Autodesk Inventor part; units mm, degrees
ref_plane "Plano inicial" through (0, 0, 35) normal (0, 0, 1) x (1, 0, 0)
ref_plane "Plano final" through (0, 0, 465) normal (0, 0, 1) x (1, 0, 0)
ref_plane "Plano de trabajo4" through (-640, 29, 465) normal (0, 0, 1) x (1, 0, 0)
ref_plane "Plano inicial" through (0, 0, 35) normal (0, 0, 1) x (1, 0, 0)
ref_plane "Plano final" through (0, 0, 465) normal (0, 0, 1) x (1, 0, 0)
sketch "Boceto" plane through (0, 0, 0) normal (0, 0, 1) x (1, 0, 0)
  line L0 (-25, -21) -> (-25, 21)
  line L1 (-21, 25) -> (21, 25)
  line L2 (25, 21) -> (25, -21)
  line L3 (21, -25) -> (-21, -25)
  arc A0 (-25, -21) -> (-21, -25) centre (-21, -21) ccw
  arc A1 (25, 21) -> (21, 25) centre (21, 21) ccw
  arc A2 (-21, 25) -> (-25, 21) centre (-21, 21) ccw
  arc A3 (21, -25) -> (25, -21) centre (21, -21) ccw
  arc A4 (-21, 23) -> (-23, 21) centre (-21, 21) ccw
  line L4 (-21, 23) -> (21, 23)
  arc A5 (23, 21) -> (21, 23) centre (21, 21) ccw
  line L5 (23, 21) -> (23, -21)
  arc A6 (21, -23) -> (23, -21) centre (21, -21) ccw
  line L6 (21, -23) -> (-21, -23)
  arc A7 (-23, -21) -> (-21, -23) centre (-21, -21) ccw
  line L7 (-23, -21) -> (-23, 21)
  line L8 (0, 36.1598) -> (0, -36.1598) construction
  line L9 (-36.1598, 0) -> (36.1598, 0) construction
  dimension "d7" = 4
  dimension "d9" = 50
  dimension "d11" = 50
  dimension "d12" = 2
  dimension "d15" = 25
  dimension "d16" = 25
extrude "Cuerpo" add sketch "Boceto" along normal up to surface (430 mm away) from surface at 35
sketch "Sketch3" plane through (0, 0, 0) normal (0, 0, 1) x (1, 0, 0)
  line L0 (0, 0) -> (10, 0)
ref_plane "Work Plane3" through (0, 0, 0) normal (0, -1, 0) x (1, 0, 0)
sketch "Sketch4" plane through (0, 0, 0) normal (0, -1, 0) x (1, 0, 0)
  line L0 (-2, 35) -> (12, 35)
  line L1 (-2, 465) -> (12, 465)
  dimension "d18" = 430
ref_plane "Plano de trabajo4" through (-640, 29, 465) normal (0, 0, 1) x (1, 0, 0)
split "Dividir1" plane through (-640, 29, 465) removes the side toward (0, 0, 1)
ref_plane "Plano de trabajo5" through (-640, -29, 35) normal (0, 0, -1) x (-1, 0, 0)
split "Dividir2" plane through (-640, -29, 35) removes the side toward (0, 0, -1)
equation "\"d7\" = G_IR"
equation "\"d9\" = G_W"
equation "\"d11\" = G_H"
equation "\"d12\" = G_T"
equation "\"d15\" = 0.5 * d9"
equation "\"d16\" = 0.5 * d11"
equation "\"d3\" = G_L"
equation "\"G_W\" = 50"
equation "\"G_H\" = 50"
equation "\"G_T\" = 2"
equation "\"G_IR\" = 4"
equation "\"G_L\" = d18"
equation "\"G_OFFSET_START\" = -35"
equation "\"G_OFFSET_END\" = -35"
equation "\"d13\" = -G_OFFSET_START"
equation "\"d14\" = G_OFFSET_END + B_L"
properties part number "ISO 10799-2 - 50x50x2 - 430" material "Galvanizado catalogo 1"
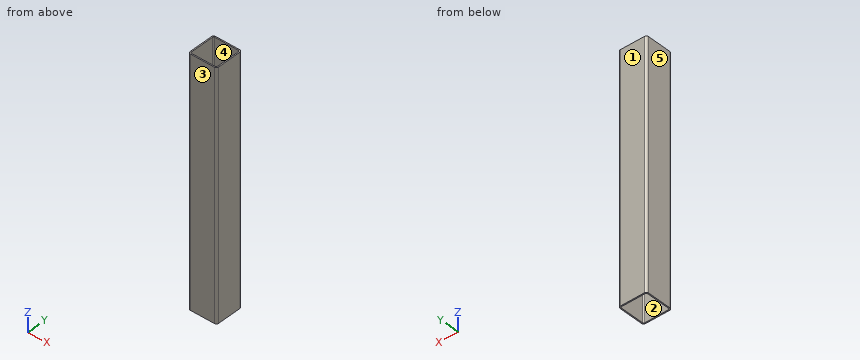
Input: part model. Units: mm. Frame: model coordinates. Face numbers are marked on the shaded views. A direction names the side the tool comes from. Round coordinates to 2 decimals unless told otherwise and drop trailing zeros. Order: outer loops, then holes, each group sorted by start corner. A loop starts at its lowest first (then second) coordinate and runs counter-clockwise, first axis right, second up. Notation, with made-up numbers: (9.25, -32.5) - (43.25, -32.5) arc R21 ccw to (43.25, -9.5) - close; hole circle Ø11 at (-15.75, 25). An arc over 180 degrees is marked (long way). Use a Markdown table: item, result.
1. Section B-B on z = 212. Return the cut outline in (x, y).
Evaluation:
| item | result |
|---|---|
| outline | (-25, -21) arc R4 ccw to (-21, -25) - (21, -25) arc R4 ccw to (25, -21) - (25, 21) arc R4 ccw to (21, 25) - (-21, 25) arc R4 ccw to (-25, 21) - close; hole (-23, -21) arc R2 ccw to (-21, -23) - (21, -23) arc R2 ccw to (23, -21) - (23, 21) arc R2 ccw to (21, 23) - (-21, 23) arc R2 ccw to (-23, 21) - close |
2. Material intervals for probe 1 along Y at (x, z) = (2.5, 88); probe 2 along Y at (x, z) = (23.5, 114), sorted ascending.
Evaluation:
| item | result |
|---|---|
| probe 1 | -25 to -23, 23 to 25 |
| probe 2 | -24.12 to 24.12 |
3. Section A-A on x = 6. Return the cut outline in (y, z).
Evaluation:
| item | result |
|---|---|
| outline | (-25, 35) - (-23, 35) - (-23, 465) - (-25, 465) - close; (23, 35) - (25, 35) - (25, 465) - (23, 465) - close |
4. Access query for the marked faces 1 and 2. Directions: +Z, -Z, +X, -X, +Y, -Y. A direction counts if a zero-diameter tool reaches every point of the face in a straight line with its end or side. Return the directions, or none.
Evaluation:
| item | result |
|---|---|
| face 1 | +Z, -Z, +X, -X, +Y |
| face 2 | +Z, -Z |
5. Mould query, pull axis X, two halves, no side actions, for the marked faces 3, 4 and 5. Classes: +X half, -X half, draft (parallel to the pull), parting line (faces both ways), or undercut.
Evaluation:
| item | result |
|---|---|
| face 3 | draft |
| face 4 | undercut |
| face 5 | -X half |
